Here's how the part is built. I have some questions about the finished solid (model axes, mm). Face numbers are marked on the shaded views. A direction names the side the tool comes from. Give positions to 0.01 mm unless a question says otherwise; leave off trailing zeros. Loops run counter-clockwise (first coordinate to the right, second up) from the corner with the lowest first, then second, coordinate; pieces in that order, holes last. Notation, with made-up numbers: (-6, 71.5) - (34, 71.5) arc R22 ccw to (34, 78.5) - close; hole circle Ø3 at (31, -37). An arc over 180 degrees is marked (long way). Return JSON: item names as keys, results as strings. Group by question number.
(1) If we section it at C-C (y = 26): Please give me the cut outline in (x, z), then the cut area to 3 significant figures.
(2) On a 3-axis mill with a long thin cutter (end or side, diameter ignored), from which of +Z, -Z, +X, -X, +Y, -Y can I reach the whole of each face in a straight line? I mean the marked faces 4, 5, 6 and 7. Say none if no direction works.
(3) If we section it at B-B (y = 49): Please give me the cut outline in (x, z).
(4) If we mould it in two halves opening along Z, with no side actions, what happens to the marked faces 1, 2 and 3? For each: released by +Z, released by -Z, zero draft, split by the parting line, or undercut.
(5) For P1, Ø10, axis at y = 36, z = 73.5, coming from the -X side; P2, Ø3, axis at x = 138, z = -70, coming from the +Y side; P3, Ø8, axis at y = 20, z = 29.5, coming from the +X side, each with a flat end and sliding along its axis, tell me the tip position at first contact or that it passes through.
(6) If we section it at A-A (x = 34.5): Please give me the cut outline in (y, z).
(7) I need wall thicknesses on probe 1 along Z at (x, y) = (190, 24); probe 2 along X at (y, z) = (34, 70); probe 3 along Z at (x, y) = (138, 52.5). Which ranges of each line are inside material? Lowest first, please. Write a range as [from, to].
(8) If we section it at D-D (z = -41): Please give me the cut outline in (x, y).
```python
from build123d import *

# Parameters (mm, degrees)
SKETCH_W         = 32
SKETCH_H         = 21.5
PAD_DEPTH        = 80
SKETCH001_W      = 70
SKETCH001_H      = 120
SKETCH001_W_2    = 140
POCKET_DEPTH     = 61.501
FILLET_R         = 10
HOLE_D           = 3.5
HOLE_CBORE_D     = 6
HOLE_CBORE_DEPTH = 15
POCKET001_DEPTH  = 15


with BuildPart() as part:
    # Sketch → Pad (new body, symmetric)
    with BuildSketch(Plane.XY):
        Polygon((0, 0), (200, 0), (200, 61.5), (128, 61.5), (128, 20), (0, 20), align=None)
        with Locations((164, 30.75)):
            Rectangle(SKETCH_W, SKETCH_H, mode=Mode.SUBTRACT)
    extrude(amount=PAD_DEPTH, both=True)

    # Sketch001 → Pocket (cut, through all)
    with BuildSketch(Plane.XZ):
        with Locations((55, 0)):
            Rectangle(SKETCH001_W, SKETCH001_H)
        with Locations((180, 0)):
            Rectangle(SKETCH001_W_2, SKETCH001_H)
    extrude(amount=-POCKET_DEPTH, mode=Mode.SUBTRACT)

    # Fillet
    fillet_edges = [part.edges().sort_by_distance(p)[0] for p in [
        (20, 10, -60),
        (0, 10, 80),
        (20, 10, 60),
        (0, 10, -80),
        (200, 0, 70),
        (200, 61.5, 70),
        (200, 61.5, -70),
        (200, 0, -70),
        (128, 61.5, 70),
        (128, 61.5, -70),
        (128, 20, 70),
        (128, 20, -70),
        (90, 10, 60),
        (90, 10, -60),
    ]]
    fillet(fillet_edges, radius=FILLET_R)

    # Hole (through all)
    with Locations(Plane(origin=(0, 61.5, 0), x_dir=(-1, 0, 0), z_dir=(0, 1, 0))):
        with Locations((-190, 70), (-138, 70), (-190, -70), (-138, -70)):
            CounterBoreHole(HOLE_D / 2, HOLE_CBORE_D / 2, HOLE_CBORE_DEPTH)

    # Sketch004 → Pocket001 (cut)
    with BuildSketch(Plane.XZ):
        Polygon((141.464102, -70), (139.732051, -67), (136.267949, -67), (134.535898, -70), (136.267949, -73), (139.732051, -73), align=None)
        Polygon((188.267949, -73), (191.732051, -73), (193.464102, -70), (191.732051, -67), (188.267949, -67), (186.535898, -70), align=None)
        Polygon((139.732051, 67), (141.464102, 70), (139.732051, 73), (136.267949, 73), (134.535898, 70), (136.267949, 67), align=None)
        Polygon((188.267949, 67), (191.732051, 67), (193.464102, 70), (191.732051, 73), (188.267949, 73), (186.535898, 70), align=None)
    extrude(amount=-POCKET001_DEPTH, mode=Mode.SUBTRACT)


solid = part.part
```
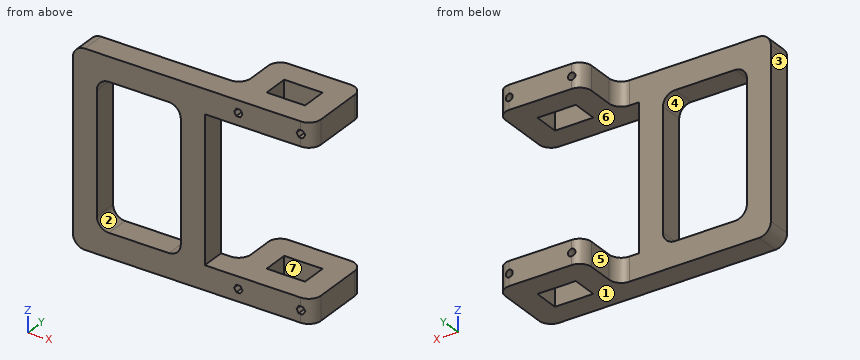
Values:
{
 "1": {"outline": "(127.17, -80) - (148, -80) - (148, -60) - (127.17, -60) - close; (127.17, 60) - (148, 60) - (148, 80) - (127.17, 80) - close; (180, -80) - (200, -80) - (200, -60) - (180, -60) - close; (180, 60) - (200, 60) - (200, 80) - (180, 80) - close; hole circle Ø3.5 at (138, -70); hole circle Ø3.5 at (138, 70); hole circle Ø3.5 at (190, -70); hole circle Ø3.5 at (190, 70)", "area": "1,590 mm2"},
 "2": {"face 4": "+Y, -Y", "face 5": "+Z, -Z, -X, +Y", "face 6": "+X, +Y, -Y", "face 7": "+Z, -Z"},
 "3": {"outline": "(128, -80) - (200, -80) - (200, -60) - (128, -60) - close; (128, 60) - (200, 60) - (200, 80) - (128, 80) - close; hole circle Ø6 at (138, -70); hole circle Ø6 at (138, 70); hole circle Ø6 at (190, -70); hole circle Ø6 at (190, 70)"},
 "4": {"face 1": "released by -Z", "face 2": "undercut", "face 3": "zero draft"},
 "5": {"P1": "x = 128", "P2": "through", "P3": "x = 110"},
 "6": {"outline": "(0, -80) - (20, -80) - (20, -60) - (0, -60) - close; (0, 60) - (20, 60) - (20, 80) - (0, 80) - close"},
 "7": {"probe 1": "[-80, -71.75], [-68.25, -60], [60, 68.25], [71.75, 80]", "probe 2": "[128, 136.25], [139.75, 148], [180, 188.25], [191.75, 200]", "probe 3": "[-80, -73], [-67, -60], [60, 67], [73, 80]"},
 "8": {"outline": "(0, 0) - (20, 0) - (20, 20) - (0, 20) - close; (90, 0) - (110, 0) - (110, 20) - (90, 20) - close"}
}
